from build123d import *

# Parameters (mm, degrees)
F1_DEPTH  = 34.29
F2_DEPTH  = 36.068
F3_DEPTH  = 89.916
F4_DEPTH  = 297.18
F5_DEPTH  = 490.22
F7_DEPTH  = 25.4
F8_DEPTH  = 25.4
F9_R      = 267.1036956646
F10_DEPTH = 25.4
F11_R     = 394.725466742
F12_DEPTH = 25.4


with BuildPart() as f1:
    # F0 (on Top) → F1 (new body)
    with BuildSketch(Plane.XY):
        with BuildLine():
            ThreePointArc((-22.0894133395, 47.1940784517), (-22.5272575475, 18.5898560115), (-50.5285451852, 12.7314313437))
            ThreePointArc((-50.5285451852, 12.7314313437), (-22.4090369372, -47.0431534459), (41.7246328393, -31.2134303949))
            ThreePointArc((41.7246328393, -31.2134303949), (19.2126905803, 0), (41.7246328393, 31.2134303949))
            ThreePointArc((41.7246328393, 31.2134303949), (12.6582281257, 50.5469334709), (-22.0894133395, 47.1940784517))
        make_face()
    extrude(amount=F1_DEPTH)

    # F2 (add): a face of the model
    f2_faces = [f1.faces().sort_by_distance(p)[0] for p in [
        (-4.6967293791, -3.1263412286, 34.29),
    ]]
    extrude(f2_faces, amount=F2_DEPTH)

    # F3 (add): a face of the model
    f3_faces = [f1.faces().sort_by_distance(p)[0] for p in [
        (-4.6967293791, -3.1263412286, 70.358),
    ]]
    extrude(f3_faces, amount=F3_DEPTH)

    # F4 (add): a face of the model
    f4_faces = [f1.faces().sort_by_distance(p)[0] for p in [
        (-4.6967293791, -3.1263412286, 160.274),
    ]]
    extrude(f4_faces, amount=F4_DEPTH)

    # F5 (add): a face of the model
    f5_faces = [f1.faces().sort_by_distance(p)[0] for p in [
        (-4.6967293791, -3.1263412286, 0),
    ]]
    extrude(f5_faces, amount=F5_DEPTH)

    # F6 (on Right) → F7 (join)
    with BuildSketch(Plane.YZ):
        Polygon((-226.492524147, -22.241378203), (-329.5620381832, -22.241378203), (-329.5620381832, -67.7837207913), (363.1609678268, -67.7837207913), (363.1609678268, 37.6827605069), (-226.492524147, 37.6827605069), align=None)
    extrude(amount=F7_DEPTH)

    # F8 (add): faces of the model
    f8_faces = [f1.faces().sort_by_distance(p)[0] for p in [
        (25.4, -164.0280914182, -20.9640918351),
        (25.4, 204.3294576408, -15.0504801422),
    ]]
    extrude(f8_faces, amount=F8_DEPTH)

    # F9 (on Right) → F10 (join)
    with BuildSketch(Plane.YZ):
        Circle(F9_R)
    extrude(amount=F10_DEPTH)

    # F11 (on Right) → F12 (join)
    with BuildSketch(Plane.YZ):
        Circle(F11_R)
    extrude(amount=F12_DEPTH)


solid = f1.part
Read the model definition and answer for the solid it produces. Units are mm, in the model's axes. A direction names the side the tool comes from. Round coordinates to 2 decimals unless told otherwise and drop trailing zeros. Write each loop counter-clockwise with the first axis right and the second up, starting at its lowest first coordinate (ties: lowest second). Pieces come first, ordered by that corner, then holes.
1. Which of the six approach directions +Z, -Z, +X, -X, +Y, -Y give full straight-line access (tool end or side, diameter ignored) to faces 5 (the face through (0, 183, 5)), 6 (the face through (38, 202, -67.784)), 7 (the face through (38, -135, 37.683))?
2. The part is cut by section C-C, the plane z = -298. Determine the outline of the cut face in (x, y).
3. The part is cut by section A-A, the plane z = 92. Determine the outline of the cut face in (x, y).
4. The part is cut by section B-B, the plane y = -203.5. Determine the outline of the cut face in (x, z).
5. Given pin 1 Ø6 at (x, z) = (6.5, 334.5) entering from -Y; pin 2 Ø12 at (x, y) = (21, 250) entering from +Z; pin 3 Ø7.5 at (x, y) = (40, 216) entering from -Z, each flat-ended and moving along its own axis, determine where each tip first touches the part or whether it passes through.
6. Straight lines are drawn through the part: L1, parallel to Y at x = 44.5, z = -5; L2, parallel to X at y = 215, z = -109; L3, parallel to Y at x = 40, z = 281.5. For each, find the intervals that lie inside material, in ascending order.
7. Determine the mould class of faces 1 (the face through (50.8, -158, -14)), 2 (the face through (12.522, -394.644, 8.042)), 3 (the face through (38, -45.498, -16)), 4 (the face through (-22.255, 18.926, -9.749)) for opening direction Y: pulls with the +Y half, pulls with the -Y half, needs draft (parallel to the pull), parting line crosses it, or undercut.
8. The part is cut by section D-D, the plane y = 171. Determine the outline of the cut face in (x, z).
Values:
1. face 5: +Z, -Z, -X, +Y
1. face 6: -Z, +X, +Y
1. face 7: +Z, +X, -Y
2. outline: (-50.53, 12.73) arc R52.11 ccw to (0, -52.11) - (0, -258.85) - (25.4, -258.85) - (25.4, -45.5) arc R52.11 ccw to (41.72, -31.21) arc R32.9 cw to (25.4, -19.2) - (25.4, 19.2) arc R32.9 cw to (41.72, 31.21) arc R52.11 ccw to (25.4, 45.5) - (25.4, 258.85) - (0, 258.85) - (0, 52.11) arc R52.11 ccw to (-22.09, 47.19) arc R22.9 cw to start
3. outline: (-50.53, 12.73) arc R52.11 ccw to (0, -52.11) - (0, -383.85) - (25.4, -383.85) - (25.4, -45.5) arc R52.11 ccw to (41.72, -31.21) arc R32.9 cw to (25.4, -19.2) - (25.4, 19.2) arc R32.9 cw to (41.72, 31.21) arc R52.11 ccw to (25.4, 45.5) - (25.4, 383.85) - (0, 383.85) - (0, 52.11) arc R52.11 ccw to (-22.09, 47.19) arc R22.9 cw to start
4. outline: (0, -338.22) - (25.4, -338.22) - (25.4, -67.78) - (50.8, -67.78) - (50.8, 37.68) - (25.4, 37.68) - (25.4, 338.22) - (0, 338.22) - close
5. pin 1: stops at y = -214.28
5. pin 2: stops at z = 310.28
5. pin 3: stops at z = -67.78
6. L1: y = -226.49 to -45.5, 45.5 to 363.16
6. L2: x = 0 to 25.4
6. L3: y = -33.39 to -30.59, 30.59 to 33.39
7. face 1: needs draft
7. face 2: pulls with the -Y half
7. face 3: undercut
7. face 4: undercut
8. outline: (0, -355.76) - (25.4, -355.76) - (25.4, -67.78) - (50.8, -67.78) - (50.8, 37.68) - (25.4, 37.68) - (25.4, 355.76) - (0, 355.76) - close
